Work out the finished part from the listing and answer in its coordinate system (mm). A direction names the side the tool comes from. Coordinates: 2 decimals unless noted, no trailing zeros. Order: outer loops, then holes, each group sorted by start corner. A loop starts at its lowest first (then second) coordinate and runs counter-clockwise, first axis right, second up. Notation, with made-up numbers: M -31,64 L 25,64 A20 ccw 25,92 Z; hole C 79,-3 d4. An arc over 180 degrees is marked long. Use a Markdown table: item, result.
from build123d import *

# Parameters (mm, degrees)
F1_DEPTH = 63.5
F2_DEPTH = 25.4
F3_DEPTH = 7.9375
F0_W     = 28.7093819976
F0_H     = 28.575
F5_R     = 6.35


with BuildPart() as f1:
    # F0 (on Front) → F1 (new body, symmetric)
    with BuildSketch(Plane.XZ):
        Polygon((41.275, -9.525), (41.275, 9.525), (22.225, 9.525), (-41.275, 9.525), (-41.275, -9.525), align=None)
    extrude(amount=F1_DEPTH, both=True)

    # F0 (on Front) → F2 (join, symmetric)
    with BuildSketch(Plane.XZ):
        with BuildLine():
            Line((22.225, 9.525), (41.275, 9.525))
            Line((41.275, 9.525), (41.275, 27.0002))
            ThreePointArc((41.275, 27.0002), (45.9246798487, 38.2255201513), (57.15, 42.8752))
            Line((57.15, 42.8752), (60.325, 42.8752))
            Line((60.325, 42.8752), (60.325, 61.9252))
            Line((60.325, 61.9252), (57.15, 61.9252))
            ThreePointArc((57.15, 61.9252), (32.4542956671, 51.6959043329), (22.225, 27.0002))
            Line((22.225, 27.0002), (22.225, 9.525))
        make_face()
        Polygon((60.325, 61.9252), (60.325, 42.8752), (60.325, 38.1), (82.4156180024, 38.1), (82.4156180024, 66.675), (60.325, 66.675), align=None)
    extrude(amount=F2_DEPTH, both=True)

    # F0 (on Front) → F3 (join, symmetric)
    with BuildSketch(Plane.XZ):
        with BuildLine():
            Line((-41.275, 9.525), (22.225, 9.525))
            Line((22.225, 9.525), (22.225, 27.0002))
            ThreePointArc((22.225, 27.0002), (32.4542956671, 51.6959043329), (57.15, 61.9252))
            add(Edge.make_bspline(
                [(-41.275, 9.525), (-40.8948995173, 39.7248640656), (9.798577653, 63.5863382701), (57.15, 61.9252)],
                knots=[0, 0, 0, 0, 111.5045361635, 111.5045361635, 111.5045361635, 111.5045361635], degree=3))
        make_face()
    extrude(amount=F3_DEPTH, both=True)

    # F0 (on Front) → F4 (revolve)
    with BuildSketch(Plane.XZ):
        with Locations((96.7703090012, 52.3875)):
            Rectangle(F0_W, F0_H)
    revolve(axis=Axis((82.4156180024, 0, 52.3875), (0, 0, 1)))

    # F5
    f5_edges = [f1.edges().sort_by_distance(p)[0] for p in [
        (-41.275, -63.5, 0),
        (41.275, -63.5, 0),
        (41.275, 63.5, 0),
        (-41.275, 63.5, 0),
    ]]
    fillet(f5_edges, radius=F5_R)


solid = f1.part
(1) A cutting plane is placed at A-A (z = -2.5). Determine the outline of the cut face in (x, y) (3 decimals).
Conclusion:
| item | result |
|---|---|
| outline | M -41.275,-57.15 A6.35 ccw -34.925,-63.5 L 34.925,-63.5 A6.35 ccw 41.275,-57.15 L 41.275,57.15 A6.35 ccw 34.925,63.5 L -34.925,63.5 A6.35 ccw -41.275,57.15 Z |
(2) A cutting plane is placed at C-C (y = -33). Determine the outline of the cut face in (x, z) (3 decimals), then the cut area to 3 significant figures.
Conclusion:
| item | result |
|---|---|
| outline | M -41.275,-9.525 L 41.275,-9.525 L 41.275,9.525 L -41.275,9.525 Z |
| area | 1,570 mm2 |
(3) Which of the six approach directions +Z, -Z, +X, -X, +Y, -Y give full straight-line access (tool end or side, diameter ignored) to faces 1 (the cylindrical face through (32.73, 16.55, 51.97)), 2 (the flat face through (22.225, -17, 18)), 3 (the flat face through (83, 0, 38.1)), 4 (the flat face through (0, -63.5, 0)), 5 (the cylindrical face through (53.708, 0.278, 40.521))?
Conclusion:
| item | result |
|---|---|
| face 1 | +Z, -X, +Y |
| face 2 | +Z, -X, -Y |
| face 3 | -Z, +X, +Y, -Y |
| face 4 | +Z, -Z, +X, -X, -Y |
| face 5 | -Z |
(4) Straight lines are drawn through the part: L1, parallel to Z at x = 101.5, y = -4.5 (3 decimals); L2, parallel to X at y = -27, z = -1.5 (3 decimals); L3, parallel to X at y = -12, z = 21 (3 decimals). For each, find the intervals that lie inside material, in ascending order.
Conclusion:
| item | result |
|---|---|
| L1 | 38.1 to 66.675 |
| L2 | -41.275 to 41.275 |
| L3 | 22.225 to 41.275 |
(5) Given P1, Ø1.6, axis at x = 58.5, y = 20, coming from the +Z side; P2, Ø6, axis at x = 29.5, z = 44.5, coming from the -Y side; P3, Ø8, axis at x = 15, z = 44, coming from the -Y side, each flat-ended and moving along its own axis, determine where each tip first touches the part or whether it passes through.
Conclusion:
| item | result |
|---|---|
| P1 | z = 61.93 |
| P2 | y = -25.4 |
| P3 | y = -7.94 |
(6) A cutting plane is placed at B-B (x = 63). Determine the outline of the cut face in (y, z) (3 decimals).
Conclusion:
| item | result |
|---|---|
| outline | M -25.4,38.1 L 25.4,38.1 L 25.4,66.675 L -25.4,66.675 Z |
